Part model, mm, in its own coordinate system. Face numbers are marked on the shaded views. A direction names the side the tool comes from. Give positions to 0.01 mm unless a question says otherwise; leave off trailing zeros. Order: outer loops, then holes, each group sorted by start corner. A loop starts at its lowest first (then second) coordinate and runs counter-clockwise, first axis right, second up. Notation, with made-up numbers: M 43.25,79 L 61.25,79 A9 cw 61.25,88 Z; hole C 53.5,76.25 d8. An arc over 180 degrees is marked long. Return JSON: item names as keys, results as strings.
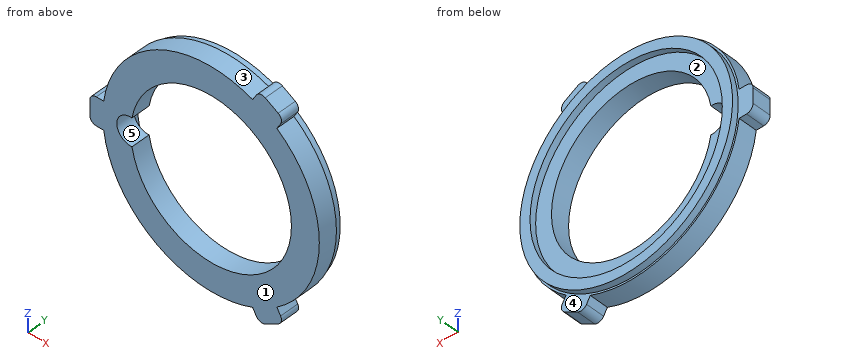
from build123d import *

# Parameters (mm, degrees)
SKIZZE1_R                       = 5.8
AUFSATZ_LINEAR_AUSTRAGEN1_DEPTH = 1
SKIZZE1_3_W                     = 1.261937381
SKIZZE1_3_H                     = 1.5
AUFSATZ_LINEAR_AUSTRAGEN2_DEPTH = 1
SKIZZE4_R                       = 4.304974062
SCHNITT_LINEAR_AUSTRAGEN1_DEPTH = 1
SKIZZE5_R                       = 0.747652737
SCHNITT_LINEAR_AUSTRAGEN2_DEPTH = 1
KREISMUSTER1_COUNT              = 3
VERRUNDUNG2_R                   = 0.35
SKIZZE6_R                       = 5.7
SKIZZE6_R_2                     = 5.1526268
AUFSATZ_LINEAR_AUSTRAGEN3_DEPTH = 0.33


with BuildPart() as part:
    # Skizze1 → Aufsatz-Linear austragen1 (new body)
    with BuildSketch(Plane(origin=(0, 0, 0), x_dir=(1, 0, 0), z_dir=(0, 1, 0))):
        Circle(SKIZZE1_R)
    extrude(amount=AUFSATZ_LINEAR_AUSTRAGEN1_DEPTH)

    # Skizze1<3> → Aufsatz-Linear austragen2 (add)
    with BuildSketch(Plane(origin=(0, 0, 0), x_dir=(1, 0, 0), z_dir=(0, 1, 0))):
        with Locations((-5.86903131, 0)):
            Rectangle(SKIZZE1_3_W, SKIZZE1_3_H)
    aufsatz_linear_austragen2 = extrude(amount=AUFSATZ_LINEAR_AUSTRAGEN2_DEPTH)

    # Skizze4 → Schnitt-Linear austragen1 (cut)
    with BuildSketch(Plane(origin=(0, 1, 0), x_dir=(1, 0, 0), z_dir=(0, 1, 0))):
        Circle(SKIZZE4_R)
    extrude(amount=-SCHNITT_LINEAR_AUSTRAGEN1_DEPTH, mode=Mode.SUBTRACT)

    # Skizze5 → Schnitt-Linear austragen2 (cut)
    with BuildSketch(Plane(origin=(0, 1, 0), x_dir=(1, 0, 0), z_dir=(0, 1, 0))):
        with Locations((-4.304974062, 0)):
            Circle(SKIZZE5_R)
    extrude(amount=-SCHNITT_LINEAR_AUSTRAGEN2_DEPTH, mode=Mode.SUBTRACT)

    # Kreismuster1: Aufsatz-Linear austragen2 ×3 about axis
    kreismuster1_axis = Axis((0, 0, 0), (0, 1, 0))
    for i in range(1, KREISMUSTER1_COUNT):
        add(aufsatz_linear_austragen2.rotate(kreismuster1_axis, i * 360 / KREISMUSTER1_COUNT))

    # Verrundung2
    verrundung2_edges = [part.edges().sort_by_distance(p)[0] for p in [
        (-6.5, 0.5, 0.75),
        (-6.5, 0.5, -0.75),
        (3.899519053, 0.5, 5.254165125),
        (2.600480947, 0.5, 6.004165125),
        (2.600480947, 0.5, -6.004165125),
        (3.899519053, 0.5, -5.254165125),
    ]]
    fillet(verrundung2_edges, radius=VERRUNDUNG2_R)

    # Skizze6 → Aufsatz-Linear austragen3 (add)
    with BuildSketch(Plane(origin=(0, 1, 0), x_dir=(1, 0, 0), z_dir=(0, 1, 0))):
        Circle(SKIZZE6_R)
        Circle(SKIZZE6_R_2, mode=Mode.SUBTRACT)
    extrude(amount=AUFSATZ_LINEAR_AUSTRAGEN3_DEPTH)


solid = part.part
Q1. Band-saw the part on C-C (y = 0.25). Give the cut face in (x, z), then the cut area to 3 significant figures.
Established:
{"outline": "M -6.5,-0.4 A0.35 ccw -6.15,-0.75 L -5.75,-0.75 A5.8 ccw 2.23,-5.36 L 2.43,-5.7 A0.35 ccw 2.9,-5.83 L 3.6,-5.43 A0.35 ccw 3.72,-4.95 L 3.53,-4.61 A5.8 ccw 3.53,4.61 L 3.72,4.95 A0.35 ccw 3.6,5.43 L 2.9,5.83 A0.35 ccw 2.43,5.7 L 2.23,5.36 A5.8 ccw -5.75,0.75 L -6.15,0.75 A0.35 ccw -6.5,0.4 Z; hole M -4.24,-0.74 A4.3 ccw long -4.24,0.74 A0.75 ccw long Z", "area": "49.6 mm²"}
Q2. Band-saw the part on A-A (z = 0). Give the cut face in (x, y).
Established:
{"outline": "M -6.5,0 L -5.05,0 L -5.05,1 L -5.15,1 L -5.15,1.33 L -5.7,1.33 L -5.7,1 L -6.5,1 Z; M 4.3,0 L 5.8,0 L 5.8,1 L 5.7,1 L 5.7,1.33 L 5.15,1.33 L 5.15,1 L 4.3,1 Z"}
Q3. 3-axis set-ups, long thin cutter, end or side, ignore diameter. For the marked faces 1 and 2: which of +Z, -Z, +X, -X, +Y, -Y reach the whole face in a straight line?
Established:
{"face 1": "+Z, -Z, +X, -X, -Y", "face 2": "+Y"}
Q4. Two-plate mould, pull along Z, no slides. Class the marked faces 3, 4 and 5: +Z half, -Z half, draft (parallel to the pull), parting line (faces both ways), or undercut.
Established:
{"face 3": "+Z half", "face 4": "draft", "face 5": "undercut"}
Q5. Probe line 1 along Z through (x, y) = (0, 1.1); line 2 along X through (y, z) = (0.7, 0); line 3 along Z through (x, y) = (0, 0.8). List the from-to ranges inside material, lowest first.
Established:
{"line 1": "z = -5.7 to -5.15, 5.15 to 5.7", "line 2": "x = -6.5 to -5.05, 4.3 to 5.8", "line 3": "z = -5.8 to -4.3, 4.3 to 5.8"}
Q6. Pin check, flat tip, straight feed: pin 1 (6 mm diameter, centred on x = 4, z = -0.5, fed in from -Y). Stop position of the tip, or through.
Established:
{"pin 1": "stops at y = 0"}
Q7. Band-saw the part on B-B (x = 0). Give the cut face in (y, z), then the cut area to 3 significant figures.
Established:
{"outline": "M 0,-5.8 L 1,-5.8 L 1,-5.7 L 1.33,-5.7 L 1.33,-5.15 L 1,-5.15 L 1,-4.3 L 0,-4.3 Z; M 0,4.3 L 1,4.3 L 1,5.15 L 1.33,5.15 L 1.33,5.7 L 1,5.7 L 1,5.8 L 0,5.8 Z", "area": "3.35 mm²"}
